Source: CAD feature listing. Evaluate the final solid. Frame: model axes, mm. A direction names the side the tool comes from. Give positions to 0.01 mm unless a question says otherwise; leave off trailing zeros. Order: outer loops, then holes, each group sorted by start corner. A loop starts at its lowest first (then second) coordinate and runs counter-clockwise, first axis right, second up. Notation, with made-up numbers: (58, 51.25) -> (113, 51.25) arc R23 ccw to (113, 85.25) -> close; hole circle Ø7 at (66, -36.5). An arc over 180 degrees is marked (long way). Answer in a Markdown table with one row per item.
```python
from build123d import *

# Parameters (mm, degrees)
SKETCH1_W            = 16
SKETCH1_H            = 16
BOSS_EXTRUDE1_DEPTH  = 9.6
SKETCH2_R            = 2.4
BOSS_EXTRUDE2_DEPTH  = 1.6
LPATTERN1_COUNT      = 2
LPATTERN1_PITCH      = 8
LPATTERN1_COUNT_DIR2 = 2
LPATTERN1_PITCH_DIR2 = 8
FILLET1_R            = 7.86
SHELL1_T             = -1.6
SKETCH3_R            = 3.256
SKETCH3_R_2          = 2.4
BOSS_EXTRUDE3_DEPTH  = 8


with BuildPart() as part:
    # Sketch1 → Boss-Extrude1 (new body)
    with BuildSketch(Plane.XY):
        with Locations((8, 8)):
            Rectangle(SKETCH1_W, SKETCH1_H)
    extrude(amount=BOSS_EXTRUDE1_DEPTH)

    # Sketch2 → Boss-Extrude2 (add)
    with BuildSketch(Plane.XY.offset(9.6)):
        with Locations(Location((4, 12, 0), (0, 0, 180))):
            Circle(SKETCH2_R)
    boss_extrude2 = extrude(amount=BOSS_EXTRUDE2_DEPTH)

    # LPattern1: Boss-Extrude2 2 × 2
    with Locations(*[(i * LPATTERN1_PITCH, -j * LPATTERN1_PITCH_DIR2, 0) for i in range(LPATTERN1_COUNT) for j in range(LPATTERN1_COUNT_DIR2) if (i, j) != (0, 0)]):
        add(boss_extrude2)

    # Fillet1
    fillet1_edges = [part.edges().sort_by_distance(p)[0] for p in [
        (0, 16, 4.8),
        (16, 16, 4.8),
        (16, 0, 4.8),
        (0, 0, 4.8),
    ]]
    fillet(fillet1_edges, radius=FILLET1_R)

    # Shell1
    shell1_openings = [part.faces().sort_by_distance(p)[0] for p in [
        (8, 8, 0),
    ]]
    offset(amount=SHELL1_T, openings=shell1_openings, kind=Kind.INTERSECTION)

    # Sketch3 → Boss-Extrude3 (add)
    with BuildSketch(Plane(origin=(0, 0, 8), x_dir=(-1, 0, 0), z_dir=(0, 0, -1))):
        with Locations((-8, 7.999999999)):
            Circle(SKETCH3_R)
        with Locations((-8, 7.999999999)):
            Circle(SKETCH3_R_2, mode=Mode.SUBTRACT)
    extrude(amount=BOSS_EXTRUDE3_DEPTH)


solid = part.part
```
(1) Access query for faces 5 (the flat face through (4, 12, 9.6)), 6 (the cylindrical face through (13.636, 2.241, 4.867)), 7 (the flat face through (8, 8, 9.6)). Directions: +Z, -Z, +X, -X, +Y, -Y. A direction counts if a zero-diameter tool reaches every point of the face in a straight line with its end or side. Return the directions, or none.
A:
| item | result |
|---|---|
| face 5 | -Z |
| face 6 | +Z, -Z, +X, -Y |
| face 7 | +Z |
(2) Section query C-C (x = 2.75). Return the cut outline in (y, z), plus the area to 3 significant figures.
A:
| item | result |
|---|---|
| outline | (1.89, 0) -> (4.24, 0) -> (4.24, 8) -> (11.76, 8) -> (11.76, 0) -> (14.11, 0) -> (14.11, 9.6) -> (14.05, 9.6) -> (14.05, 11.2) -> (9.95, 11.2) -> (9.95, 9.6) -> (6.05, 9.6) -> (6.05, 11.2) -> (1.95, 11.2) -> (1.95, 9.6) -> (1.89, 9.6) -> close |
| area | 70.4 mm^2 |
(3) First-contact query: pin 1 Ø6 at (y, z) = (13, 10) entering from -X; pin 2 Ø2 at (x, z) = (3.5, 4.5) entering from -Y; pin 3 Ø2.5 at (x, y) = (9, 7.5) entering from -Z. Flat tips, straight axial feed; report the tip coordinate or a pass-through.
A:
| item | result |
|---|---|
| pin 1 | stops at x = 0.23 |
| pin 2 | stops at y = 0.75 |
| pin 3 | stops at z = 8 |
(4) Pull-direction query (X, two-part tool) for faces 1 (the cylindrical face through (12.31, 9.62, 10.39)), 2 (the cylindrical face through (13.636, 13.759, 4.867)), 3 (the flat face through (6, 11, 8)), 4 (the flat face through (4, 4, 11.2)); classes: +X half, -X half, draft (parallel to the pull), parting line (faces both ways), or undercut.
A:
| item | result |
|---|---|
| face 1 | undercut |
| face 2 | +X half |
| face 3 | undercut |
| face 4 | draft |
(5) Section query A-A (z = 3.25). Return the cut outline in (x, y), plus the area to 3 significant figures.
A:
| item | result |
|---|---|
| outline | (0, 7.86) arc R7.86 ccw to (7.86, 0) -> (8.14, 0) arc R7.86 ccw to (16, 7.86) -> (16, 8.14) arc R7.86 ccw to (8.14, 16) -> (7.86, 16) arc R7.86 ccw to (0, 8.14) -> close; circle Ø6.51 at (8, 8); hole (1.6, 7.86) arc R6.26 ccw to (7.86, 1.6) -> (8.14, 1.6) arc R6.26 ccw to (14.4, 7.86) -> (14.4, 8.14) arc R6.26 ccw to (8.14, 14.4) -> (7.86, 14.4) arc R6.26 ccw to (1.6, 8.14) -> close; hole circle Ø4.8 at (8, 8) |
| area | 88.0 mm^2 |
(6) Section query B-B (z = 8.75). Return the cut outline in (x, y), plus the area to 3 significant figures.
A:
| item | result |
|---|---|
| outline | (0, 7.86) arc R7.86 ccw to (7.86, 0) -> (8.14, 0) arc R7.86 ccw to (16, 7.86) -> (16, 8.14) arc R7.86 ccw to (8.14, 16) -> (7.86, 16) arc R7.86 ccw to (0, 8.14) -> close; hole circle Ø1.6 at (4, 4); hole circle Ø1.6 at (4, 12); hole circle Ø1.6 at (12, 4); hole circle Ø1.6 at (12, 12) |
| area | 195 mm^2 |
(7) Section query D-D (y = 11.5). Return the cut outline in (x, z), plus the area to 3 significant figures.
A:
| item | result |
|---|---|
| outline | (0.75, 0) -> (2.58, 0) -> (2.58, 8) -> (3.38, 8) -> (3.38, 9.6) -> (4.62, 9.6) -> (4.62, 8) -> (11.38, 8) -> (11.38, 9.6) -> (12.62, 9.6) -> (12.62, 8) -> (13.42, 8) -> (13.42, 0) -> (15.25, 0) -> (15.25, 9.6) -> (14.35, 9.6) -> (14.35, 11.2) -> (9.65, 11.2) -> (9.65, 9.6) -> (6.35, 9.6) -> (6.35, 11.2) -> (1.65, 11.2) -> (1.65, 9.6) -> (0.75, 9.6) -> close |
| area | 63.4 mm^2 |
(8) Ray query, probe 1 along X at (y, z) = (8, 4.75); probe 2 along Y at (x, z) = (10.5, 4.25). Return the intervals inside material, ascending.
A:
| item | result |
|---|---|
| probe 1 | x = 0 to 1.6, 4.74 to 5.6, 10.4 to 11.26, 14.4 to 16 |
| probe 2 | y = 0.36 to 2.06, 5.91 to 10.09, 13.94 to 15.64 |
